Autodesk Inventor part; units mm, degrees
ref_plane "YZ Plane" through (0, 0, 0) normal (1, 0, 0) x (0, 1, 0)
ref_plane "XZ Plane" through (0, 0, 0) normal (0, 1, 0) x (-1, 0, 0)
ref_plane "XY Plane" through (0, 0, 0) normal (0, 0, 1) x (1, 0, 0)
sketch "Esboço1" plane through (0, 0, 0) normal (0, 0, 1) x (1, 0, 0)
  circle A0 centre (0, 0) radius 5
  dimension "d0" = 10
extrude "Extrusão1" add sketch "Esboço1" along normal blind 1
sketch "Esboço2" plane through (0, 0, 1) normal (0, 0, 1) x (1, 0, 0)
  circle A0 centre (0, 0) radius 4
  dimension "d3" = 8
extrude "Extrusão2" add sketch "Esboço2" along normal blind 1
sketch "Esboço3" plane through (0, 0, 2) normal (0, 0, 1) x (1, 0, 0)
  circle A0 centre (0, 0) radius 5
  dimension "d6" = 10
extrude "Extrusão3" add sketch "Esboço3" along normal blind 1
sketch "Esboço4" plane through (0, 0, 3) normal (0, 0, 1) x (1, 0, 0)
  circle A0 centre (0, 0) radius 4
  circle A1 centre (0, 0) radius 1
  dimension "d9" = 2
extrude "Extrusão4" cut sketch "Esboço4" against normal blind 4 contours A1
thread "Rosca1"
sketch "Esboço5" plane through (0, 0, 3) normal (0, 0, 1) x (1, 0, 0)
  circle A0 centre (0, 0) radius 5
  line L0 (-4, 0) -> (-4, -0.5)
  circle A1 centre (0, 0) radius 4
  line L1 (-4, 0) -> (-3.5, 0) construction
  line L2 (-4, -0.5) -> (-5, -0.5)
  line L3 (-5, -0.5) -> (-5, 0.5)
  line L4 (-5, -0.5) -> (-4, -0.5) construction
  line L5 (-5, 0.5) -> (-4, 0.5)
  line L6 (-4, 0.5) -> (-4, 0)
  line L7 (-4, -0.5) -> (-5, -0.5)
  dimension "d15" = 0.5
  dimension "d16" = 90
  dimension "d17" = 1
  dimension "d18" = 90
extrude "Extrusão5" cut sketch "Esboço5" against normal blind 10 contours L5 L6 L0 L2 A0 | A0 L3 L5 | L2 L3 A0 picked at (-4.3296, -0.2779)
properties part number "Polia"
Geometry check sheet. Reference: the model listing, model coordinates, mm. A direction names the side the tool comes from. Give positions to 0.01 mm unless a question says otherwise; leave off trailing zeros. Order: outer loops, then holes, each group sorted by start corner. A loop starts at its lowest first (then second) coordinate and runs counter-clockwise, first axis right, second up. Notation, with made-up numbers: (30.25, 15.25) - (67.25, 15.25) arc R17 cw to (67.25, 28.25) - close; hole circle Ø11 at (-6.5, -9.5). An arc over 180 degrees is marked (long way). Answer in a Markdown table with one row per item. Add a question column.
Q1. Material ranges on probe 1 along Z at (x, y) = (3.5, -3.5); probe 2 along Y at (x, z) = (0, 0.95); probe 3 along Y at (x, z) = (0, 1.2), recorded low to high. Write a range as from..to.
Q2. Cross-section at D-D, the plane y = -2.5. Enter the section's corners in (x, z).
Q3. Cross-section at C-C, the plane y = 4.25. Enter the section's corners in (x, z).
Q4. Gauge pin test, flat ends, axial feed: pin 1 (0.8 mm diameter, centred on x = -4.5, z = 2.5, fed in from +Y); pin 2 (0.5 mm diameter, centred on x = -4.5, z = 2.5, fed in from -Y); pin 3 (1.1 mm diameter, centred on x = -4.5, z = 0.5, fed in from -Y). Record the tip position at first contact, or that the pin passes through.
Q5. Mould release check, pull along Z, two halves, no side actions. Record for faces 1 (the flat face through (4, 2, 1)), 2 (the cylindrical face through (4.995, 0.213, 2.493)), 3 (the flat face through (-1.2, 0.1, 3)): pulls with the +Z half, pulls with the -Z half, needs draft (parallel to the pull), parting line crosses it, or undercut.
Q6. Cross-section at B-B, the plane z = 2.35. Enter the section's corners in (x, y).
Q7. Cross-section at A-A, the plane x = 0. Enter the section's corners in (y, z).
Q8. Tool access check on faces 4 (the flat face through (4, 2, 2)), 5 (the cylindrical face through (4.995, 0.213, 0.493)), 6 (the flat face through (-4.5, 0.5, 0.5)). Record the directions out of +Z, -Z, +X, -X, +Y, -Y that give a thin tool (end or side, any length) a straight path to the whole face; none if there is none.
Check values:
| question | item | result |
|---|---|---|
| 1 | probe 1 | z = 0..1, 2..3 |
| 1 | probe 2 | y = -5..-1, 1..5 |
| 1 | probe 3 | y = -4..-1, 1..4 |
| 2 | outline | (-4.33, 0) - (4.33, 0) - (4.33, 1) - (3.12, 1) - (3.12, 2) - (4.33, 2) - (4.33, 3) - (-4.33, 3) - (-4.33, 2) - (-3.12, 2) - (-3.12, 1) - (-4.33, 1) - close |
| 3 | outline | (-2.63, 0) - (2.63, 0) - (2.63, 1) - (-2.63, 1) - close; (-2.63, 2) - (2.63, 2) - (2.63, 3) - (-2.63, 3) - close |
| 4 | pin 1 | stops at y = 2.86 |
| 4 | pin 2 | stops at y = -2.63 |
| 4 | pin 3 | stops at y = -3.07 |
| 5 | face 1 | undercut |
| 5 | face 2 | needs draft |
| 5 | face 3 | pulls with the +Z half |
| 6 | outline | (-4.97, -0.5) arc R5 ccw (long way) to (-4.97, 0.5) - (-4, 0.5) - (-4, -0.5) - close; hole circle Ø2 at (0, 0) |
| 7 | outline | (-5, 0) - (-1, 0) - (-1, 3) - (-5, 3) - (-5, 2) - (-4, 2) - (-4, 1) - (-5, 1) - close; (1, 0) - (5, 0) - (5, 1) - (4, 1) - (4, 2) - (5, 2) - (5, 3) - (1, 3) - close |
| 8 | face 4 | none |
| 8 | face 5 | +Z, -Z |
| 8 | face 6 | +Z, -Z, -X |
